Part model, mm, in its own coordinate system. A direction names the side the tool comes from. Give positions to 0.01 mm unless a question says otherwise; leave off trailing zeros. Loops run counter-clockwise (first coordinate to the right, second up) from the corner with the lowest first, then second, coordinate; pieces in that order, holes last. Notation, with made-up numbers: (-21, -4.75) -> (-2, -4.75) arc R19 ccw to (-2, 20.25) -> close; hole circle Ø2 at (42.25, 29). An arc over 180 degrees is marked (long way). One line per question, with ' | ' between items.
```python
from build123d import *

# Parameters (mm, degrees)
F3_T     = -2.54
F2_R     = 4.327006367
F4_DEPTH = 75.5575296859


with BuildPart() as f1:
    # F0 (on Top) → F1 (revolve)
    with BuildSketch(Plane.XY):
        Polygon((0, 20.3673411161), (0, -55.1891885698), (16.3254532963, -55.1891885698), (16.3254532963, -30.9031605721), (31.7451581359, -9.701074101), (31.7451581359, 20.3673411161), align=None)
    revolve(axis=Axis((0, -6.6171362996, 0), (0, -1, 0)))

    # F3
    f3_openings = [f1.faces().sort_by_distance(p)[0] for p in [
        (0, 20.367341, 0),
    ]]
    offset(amount=F3_T, openings=f3_openings, kind=Kind.INTERSECTION)

    # F2 (on face) → F4 (cut, through all)
    with BuildSketch(Plane.XZ.offset(55.1891885698)):
        Circle(F2_R)
    extrude(amount=-F4_DEPTH, mode=Mode.SUBTRACT)


solid = f1.part
```
1) Drill centre lines: line 1 (Z direction, x = 0, y = -54.55); line 2 (Z direction, x = 0, y = -41); line 3 (Y direction, x = 5.5, z = 11.5). Where is each one in solid material? Low to high.
Found:
line 1: -16.33 to -4.33, 4.33 to 16.33 | line 2: -16.33 to -13.79, 13.79 to 16.33 | line 3: -55.19 to -52.65
2) Pull direction Z, two halves, no side cores. Call faces 4 (the flat face through (14, 20.367, -26)), 5 (the cylindrical face through (-3.434, -53.937, -2.633)), 6 (the cylindrical face through (29.324, 5.544, -12.159)): pulls with the +Z half, pulls with the -Z half, needs draft (parallel to the pull), parting line crosses it, or undercut.
Found:
face 4: needs draft | face 5: undercut | face 6: parting line crosses it
3) Saw through at B-B (x = 0). Give the cut face in (y, z).
Found:
outline: (-55.19, -16.33) -> (-30.9, -16.33) -> (-9.7, -31.75) -> (20.37, -31.75) -> (20.37, -29.21) -> (-8.88, -29.21) -> (-30.08, -13.79) -> (-52.65, -13.79) -> (-52.65, -4.33) -> (-55.19, -4.33) -> close; (-55.19, 4.33) -> (-52.65, 4.33) -> (-52.65, 13.79) -> (-30.08, 13.79) -> (-8.88, 29.21) -> (20.37, 29.21) -> (20.37, 31.75) -> (-9.7, 31.75) -> (-30.9, 16.33) -> (-55.19, 16.33) -> close
4) Pin check, flat tips, straight feed: P1, Ø2, axis at x = -22, z = 20.5, coming from the -Y side; P2, Ø8.5, axis at x = 6, z = -1, coming from the +Y side; P3, Ø2, axis at y = 8, z = -4, coming from the +X side. Stop position of each tip, or through.
Found:
P1: y = -13.38 | P2: y = -52.65 | P3: x = 31.6
5) Tool access for faces 1 (the flat face through (-3.4, -55.189, -3.4)), 2 (the cylindrical face through (15.08, -42.88, -6.25)), 3 (the cylindrical face through (-6.33, 5.95, -28.51)): list every direction of +Z, -Z, +X, -X, +Y, -Y with a clear straight run to the whole face (end or side of a thin tool).
Found:
face 1: +Z, -Z, +X, -X, -Y | face 2: -Y | face 3: +Y
6) Saw through at A-A (z = 0). Give the cut face in (x, y), and give its area (3 significant figures).
Found:
outline: (-31.75, -9.7) -> (-16.33, -30.9) -> (-16.33, -55.19) -> (-4.33, -55.19) -> (-4.33, -52.65) -> (-13.79, -52.65) -> (-13.79, -30.08) -> (-29.21, -8.88) -> (-29.21, 20.37) -> (-31.75, 20.37) -> close; (4.33, -55.19) -> (16.33, -55.19) -> (16.33, -30.9) -> (31.75, -9.7) -> (31.75, 20.37) -> (29.21, 20.37) -> (29.21, -8.88) -> (13.79, -30.08) -> (13.79, -52.65) -> (4.33, -52.65) -> close | area: 457 mm2
7) Saw through at D-D (y = -18.5). Give the cut face in (x, z).
Found:
outline: circle Ø50.69 at (0, 0); hole circle Ø44.41 at (0, 0)
8) Saw through at C-C (y = 7.5). Give the cut face in (x, z).
Found:
outline: circle Ø63.49 at (0, 0); hole circle Ø58.41 at (0, 0)
